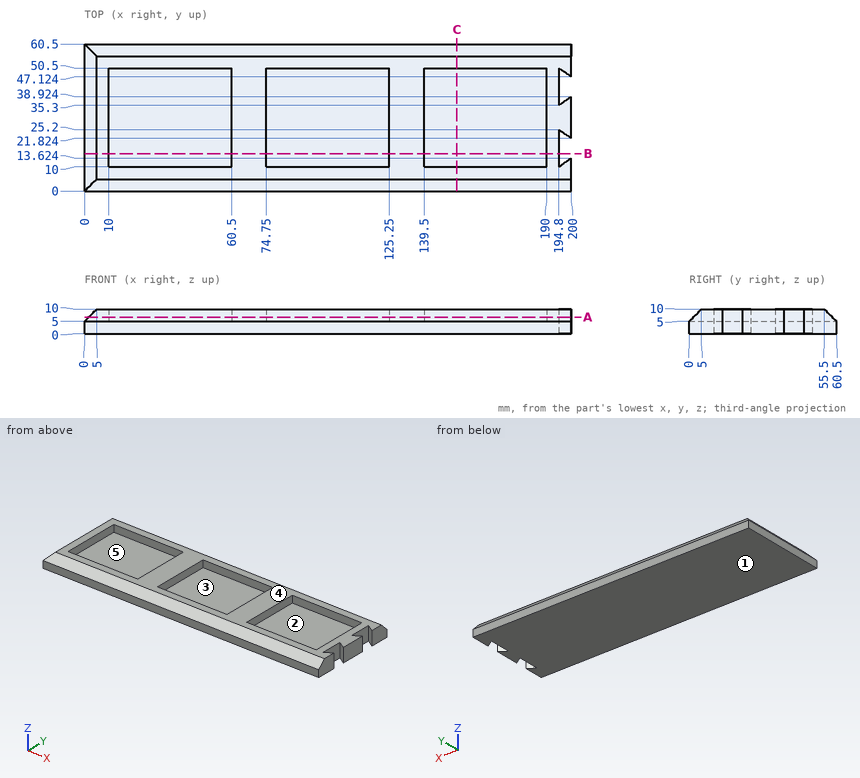
Design review of the part shown in the three views and the two pictorial views. Dimensions are in mm from the part's minimum x, y and z. A direction names the side the tool comes from. Give positions to 0.01 mm unless a question says otherwise; leave off trailing zeros. Loops run counter-clockwise (first coordinate to the right, second up) from the corner with the lowest first, then second, coordinate; pieces in that order, holes last. Notation, with made-up numbers: M 13.25,-23 L 40.25,-23 A24 ccw 40.25,13 Z; hole C 27,5.25 d2. An arc over 180 degrees is marked long. Answer as a JSON object with one key per item and string values. Group by question number.
Q1. For probe 1 along X at (y, z) = (28.5, 6.75); probe 2 along X at (y, z) = (39, 9.25); probe 3 along X at (y, z) = (23.5, 7.75), list the stretches that pass through material, from the lowest coordinate up. Write a range as [from, to].
Q2. Tool access review of the marked faces 1 and 2: name each direction out of +Z, -Z, +X, -X, +Y, -Y from which nothing blocks a thin tool from reaching the whole face with its end or side.
Q3. Insertion check: P1, Ø1, axis at x = 168.5, y = 33.5, coming from the +Z side; P2, Ø1.5, axis at y = 31.5, z = 8, coming from the -X side; P3, Ø2.5, axis at x = 34.5, z = 7, coming from the -Y side. Each pin has a flat end and moves straight along its axis. Give the tip position at first contact, or say it passes through.
Q4. Add section C-C on x = 153. Give the boundary of the cut face in (y, z).
Q5. Mouldability with a two-part tool opening along X and no side actions: class the marked faces 3, 4 and 5 as +X half, -X half, draft (parallel to the pull), parting line (faces both ways), or undercut.
Q6. Add section B-B on y = 15.5. Give the boundary of the cut face in (x, z).
Q7. Add section A-A on z = 6.75. Give the boundary of the cut face in (x, y).
Checked values:
{
 "1": {"probe 1": "[1.75, 10], [60.5, 74.75], [125.25, 139.5], [190, 200]", "probe 2": "[4.25, 10], [60.5, 74.75], [125.25, 139.5], [190, 194.8]", "probe 3": "[2.75, 10], [60.5, 74.75], [125.25, 139.5], [190, 194.8], [197.42, 200]"},
 "2": {"face 1": "-Z, +X, -X, +Y, -Y", "face 2": "+Z"},
 "3": {"P1": "z = 5", "P2": "x = 2.25", "P3": "y = 0.75"},
 "4": {"outline": "M 0,0 L 60.5,0 L 60.5,5 L 55.5,10 L 50.5,10 L 50.5,5 L 10,5 L 10,10 L 5,10 L 0,5 Z"},
 "5": {"face 3": "undercut", "face 4": "draft", "face 5": "undercut"},
 "6": {"outline": "M 0,0 L 194.8,0 L 194.8,10 L 190,10 L 190,5 L 139.5,5 L 139.5,10 L 125.25,10 L 125.25,5 L 74.75,5 L 74.75,10 L 60.5,10 L 60.5,5 L 10,5 L 10,10 L 5,10 L 0,5 Z"},
 "7": {"outline": "M 1.75,1.75 L 200,1.75 L 200,13.62 L 194.8,10 L 194.8,25.2 L 200,21.82 L 200,38.92 L 194.8,35.3 L 194.8,50.5 L 200,47.12 L 200,58.75 L 1.75,58.75 Z; hole M 10,10 L 60.5,10 L 60.5,50.5 L 10,50.5 Z; hole M 74.75,10 L 125.25,10 L 125.25,50.5 L 74.75,50.5 Z; hole M 139.5,10 L 190,10 L 190,50.5 L 139.5,50.5 Z"}
}
